Build history of the part. All positions in model axes, mm. Face numbers are marked on the shaded views. A direction names the side the tool comes from. Give positions to 0.01 mm unless a question says otherwise; leave off trailing zeros. Loops run counter-clockwise (first coordinate to the right, second up) from the corner with the lowest first, then second, coordinate; pieces in that order, holes last.
1) Wall check: line 1 (Z direction, x = 34.5, y = 23.5); line 2 (X direction, y = 30, z = 6.5). Give the ranges that are in metal, low to high.
2) Band-saw the part on C-C on z = 30. List the corners of the cut face in (x, y).
3) Flat gauge pin, fed straight in: P1, Ø10, axis at y = 36.5, z = 19, coming from the +X side. Where does the tip first touch, or does it go through?
4) 3-axis set-ups, long thin cutter, end or side, ignore diameter. For the marked faces 1 and 2: which of +Z, -Z, +X, -X, +Y, -Y reach the whole face in a straight line?
5) Band-saw the part on A-A on x = 12. List the corners of the cut face in (y, z).
6) Band-saw the part on B-B on y = 32. List the corners of the cut face in (x, z), then the cut area to 3 significant figures.
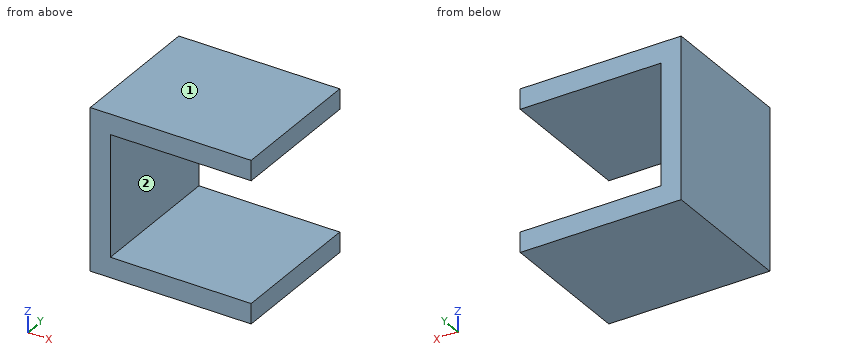
Solid Edge part; units mm, degrees
sketch "Sketch1" plane through (0, 0, 0) normal (1, 0, 0) x (0, 1, 0)
  line L0 (0, 0) -> (43.8289, 0)
sketch "Sketch2" plane through (0, 0, 0) normal (0, -1, 0) x (1, 0, 0)
  line L0 (0, 50.8) -> (0, 0)
  line L1 (0, 0) -> (50.8, 0)
  line L2 (50.8, 0) -> (50.8, 6.35)
  line L3 (50.8, 6.35) -> (6.35, 6.35)
  line L4 (6.35, 6.35) -> (6.35, 44.45)
  line L5 (6.35, 44.45) -> (50.8, 44.45)
  line L6 (50.8, 44.45) -> (50.8, 50.8)
  line L7 (50.8, 50.8) -> (0, 50.8)
sweep "SweptProtrusion_1" add profiles "Sketch2" path "Sketch1"
Findings below:
1. line 1: z = 0 to 6.35, 44.45 to 50.8
1. line 2: x = 0 to 6.35
2. outline: (0, 0) - (6.35, 0) - (6.35, 43.83) - (0, 43.83) - close
3. P1: stops at x = 6.35
4. face 1: +Z, +X, -X, +Y, -Y
4. face 2: +X, +Y, -Y
5. outline: (0, 0) - (43.83, 0) - (43.83, 6.35) - (0, 6.35) - close; (0, 44.45) - (43.83, 44.45) - (43.83, 50.8) - (0, 50.8) - close
6. outline: (0, 0) - (50.8, 0) - (50.8, 6.35) - (6.35, 6.35) - (6.35, 44.45) - (50.8, 44.45) - (50.8, 50.8) - (0, 50.8) - close
6. area: 887 mm2
